Check sheet for the modelled part. Datum: model origin and axes. Units: mm. Face numbers are marked on the shaded views. A direction names the side the tool comes from. Round coordinates to 2 decimals unless told otherwise and drop trailing zeros. Order: outer loops, then holes, each group sorted by start corner. A loop starts at its lowest first (then second) coordinate and runs counter-clockwise, first axis right, second up.
(1) Mould release check, pull along Z, two halves, no side actions. Record for the marked faces 4, 5, 6 and 7: released by +Z, released by -Z, zero draft, split by the parting line, or undercut.
(2) Tool access check on the marked faces 1, 2 and 3. Record the directions out of +Z, -Z, +X, -X, +Y, -Y that give a thin tool (end or side, any length) a straight path to the whole face; none if there is none.
(3) Thickness scan on probe 1 along Y at (x, z) = (-3.5, -3); probe 2 along X at (y, z) = (56, -0.75); probe 3 along X at (y, z) = (23.5, -1). Record the ranges inside material, lowest first.
(4) Depth check by flat-ended pin: pin 1 (3 mm diameter, centred on y = 43, z = -4, fed in from +X); pin 2 (1 mm diameter, centred on y = 22.5, z = -1, fed in from -X); pin 3 (5 mm diameter, centred on x = -3.5, y = 43, fed in from -Z); pin 4 (2 mm diameter, centred on y = 46, z = 1.5, fed in from -X). Enter the tip coordinate at first touch or a pass-through.
(5) Sectioned sample at B-B, the plane y = 38. Enter the section's corners in (x, z).
(6) Sectioned sample at A-A, the plane y = 9. Enter the section's corners in (x, z).
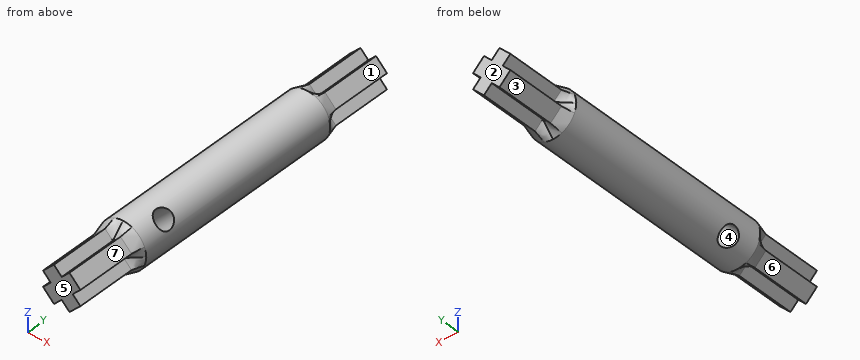
```python
from build123d import *

# Parameters (mm, degrees)
BOSS_EXTRUDE1_DEPTH = 13.804347826
SCALE1_SCALE        = 0.92
SKETCH2_R           = 4.953
SKETCH3_R           = 4.953
BOSS_EXTRUDE2_DEPTH = 22.86
BOSS_EXTRUDE4_DEPTH = 13.804347826
SCALE2_SCALE        = 0.92
SKETCH6_R           = 2.032
CUT_EXTRUDE1_DEPTH  = 78.679240568


with BuildPart() as part:
    # Sketch1 → Boss-Extrude1 (new body)
    with BuildSketch(Plane(origin=(0, 0, 0), x_dir=(1, 0, 0), z_dir=(0, 1, 0))):
        Polygon((-0.6269783, 2.91618698), (-2.423029524, 4.712238204), (-4.963029524, 2.172238204), (-3.1669783, 0.37618698), (-4.963029524, -1.419864244), (-2.423029524, -3.959864244), (-0.6269783, -2.16381302), (1.169072924, -3.959864244), (3.709072924, -1.419864244), (1.9130217, 0.37618698), (3.709072924, 2.172238204), (1.169072924, 4.712238204), align=None)
    extrude(amount=BOSS_EXTRUDE1_DEPTH)


with BuildPart() as part_1:
    # Scale1: scaled about (-0.6269783, 6.902173913, -0.37618698)
    add(part.part.scale(SCALE1_SCALE).moved(Location((-0.050158264, 0.552173913, -0.030094958))))

    # Sketch2 → section 1 of loft1
    with BuildSketch(Plane(origin=(0, 15.792173913, 0), x_dir=(1, 0, 0), z_dir=(0, 1, 0)), mode=Mode.PRIVATE) as loft1_s1:
        with Locations((-0.6269783, 0.37618698)):
            Circle(SKETCH2_R)
    # loft from a face of the part (loft1)
    loft([part_1.faces().sort_by_distance((-0.6269783, 13.252173913, -0.37618698))[0], loft1_s1.sketch])

    # Sketch3 → Boss-Extrude2 (add)
    with BuildSketch(Plane(origin=(0, 15.792173913, 0), x_dir=(1, 0, 0), z_dir=(0, 1, 0))):
        with Locations(Location((-0.6269783, 0.37618698, 0), (0, 0, 270))):
            Circle(SKETCH3_R)
    boss_extrude2 = extrude(amount=BOSS_EXTRUDE2_DEPTH)

    # Mirror6: Boss-Extrude2 across plane
    add(boss_extrude2.mirror(Plane(origin=(-0.6269783, 38.652173913, -0.37618698), x_dir=(0, 0, 1), z_dir=(0, 1, 0))))



with BuildPart() as body_2:
    # Sketch5 → Boss-Extrude4 (new body)
    with BuildSketch(Plane(origin=(0, 63.500993913, 0), x_dir=(1, 0, 0), z_dir=(0, 1, 0))):
        Polygon((-0.6269783, 2.91618698), (-2.423029524, 4.712238204), (-4.963029524, 2.172238204), (-3.1669783, 0.37618698), (-4.963029524, -1.419864244), (-2.423029524, -3.959864244), (-0.6269783, -2.16381302), (1.169072924, -3.959864244), (3.709072924, -1.419864244), (1.9130217, 0.37618698), (3.709072924, 2.172238204), (1.169072924, 4.712238204), align=None)
    extrude(amount=BOSS_EXTRUDE4_DEPTH)


with BuildPart() as body_2_1:
    # Scale2: scaled about (-0.6269783, 70.403167826, -0.37618698)
    add(body_2.part.scale(SCALE2_SCALE).moved(Location((-0.050158264, 5.632253426, -0.030094958))))


with BuildPart() as part_2:
    add(part_1.part)

    add(body_2_1.part)  # loft2 joins it to this body
    # loft from a face of the part (loft2)
    loft([part_2.faces().sort_by_distance((-0.6269783, 61.512173913, -0.37618698))[0], part_2.faces().sort_by_distance((-0.6269783, 64.053167826, -0.37618698))[0]])

    # Sketch6 → Cut-Extrude1 (cut, through all)
    with BuildSketch(Plane(origin=(-4.003882527, 0, -4.003882527), x_dir=(-0.7071067811865471, 0, 0.7071067811865479), z_dir=(-0.7071067811865479, 0, -0.7071067811865471))):
        with Locations((0.177336243, 21.888173913)):
            Circle(SKETCH6_R)
    extrude(amount=-CUT_EXTRUDE1_DEPTH, mode=Mode.SUBTRACT)


solid = part_2.part
```
Derived:
1. face 4: undercut
1. face 5: zero draft
1. face 6: released by -Z
1. face 7: released by +Z
2. face 1: +Z, +X, +Y
2. face 2: +Z, -Z, +X, -X, +Y
2. face 3: -Z, -X, +Y
3. probe 1: y = 0.55 to 19.86, 23.91 to 76.75
3. probe 2: x = -5.57 to 4.31
3. probe 3: x = -5.54 to -3, 0.5 to 4.29
4. pin 1: stops at x = 3.85
4. pin 2: stops at x = -5.58
4. pin 3: stops at z = -5.32
4. pin 4: stops at x = -5.5
5. outline: circle Ø9.91 at (-0.63, -0.38)
6. outline: (-4.62, -2.03) - (-2.28, -4.37) - (-0.63, -2.71) - (1.03, -4.37) - (3.36, -2.03) - (1.71, -0.38) - (3.36, 1.28) - (1.03, 3.61) - (-0.63, 1.96) - (-2.28, 3.61) - (-4.62, 1.28) - (-2.96, -0.38) - close
